The listing builds one solid part. Answer for the finished solid, in the listing's coordinates (mm). Face numbers are marked on the shaded views. Round coordinates to 2 decimals unless told otherwise and drop trailing zeros. Write each loop counter-clockwise with the first axis right and the second up, starting at its lowest first coordinate (ties: lowest second). Pieces come first, ordered by that corner, then holes. Notation, with made-up numbers: (-5, 67) -> (30, 67) arc R28 ccw to (30, 97) -> close; hole circle Ø3 at (-30, 44). An arc over 180 degrees is marked (long way). Write each question's results on one line, items separated by ' | '. Start each with the question number.
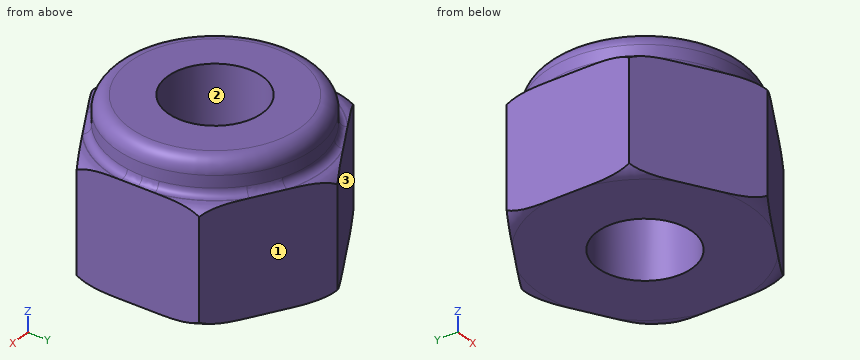
Autodesk Inventor part; units mm, degrees
ref_plane "Work Plane1" through (-12.7, 19.1158, 5.969) normal (-1, 0, 0) x (0, 0, -1)
ref_plane "YZ Plane" through (0, 0, 0) normal (1, 0, 0) x (0, 1, 0)
ref_plane "XZ Plane" through (0, 0, 0) normal (0, 1, 0) x (-1, 0, 0)
sketch "Sketch1" plane through (0, 0, 0) normal (0, 0, 1) x (1, 0, 0)
  line L0 (-12.7, 6.2842) -> (-18.2562, 9.4921)
  line L1 (-18.2562, 9.4921) -> (-18.2563, 15.9079)
  line L2 (-18.2563, 15.9079) -> (-12.7, 19.1158)
  line L3 (-12.7, 19.1158) -> (-7.1438, 15.9079)
  line L4 (-7.1438, 15.9079) -> (-7.1438, 9.4921)
  line L5 (-7.1438, 9.4921) -> (-12.7, 6.2842)
  point P0 (-12.7, 12.7)
  dimension "d0" = 11.1125
extrude "Extrusion1" add sketch "Sketch1" along normal blind 5.969
ref_plane "Work Plane1" through (-12.7, 19.1158, 5.969) normal (-1, 0, 0) x (0, 0, -1)
sketch "Sketch3" plane through (-12.7, 19.1158, 5.969) normal (-1, 0, 0) x (0, 0, -1)
  line L0 (0, 12.8316) -> (5.969, 12.8316)
  line L1 (5.969, 12.8316) -> (5.969, 0)
  line L2 (5.969, 0) -> (0, 0)
  line L3 (0, 0) -> (0, 12.8316)
  line L4 (0, 12.0696) -> (0, 6.4158)
  line L5 (0, 6.4158) -> (5.969, 6.4158)
  line L6 (5.969, 6.4158) -> (5.969, 12.0696)
  arc A0 (5.969, 12.0696) -> (5.625, 12.8316) centre (4.953, 12.0696) ccw
  arc A1 (0.344, 12.8316) -> (0, 12.0696) centre (1.016, 12.0696) ccw
  line L7 (0.344, 12.8316) -> (5.625, 12.8316)
  line L8 (5.969, 12.8316) -> (5.969, 9.6237)
  line L9 (0, 12.8316) -> (0, 9.6237)
  line L10 (0, 9.6237) -> (0, 3.2079)
  dimension "d4" = 1.016
  dimension "d5" = 0.762
  dimension "d6" = 0.762
revolve "Revolution1" cut sketch "Sketch3" angle 360 about axis through (-12.7, 12.7, 5.969) along (0, 0, -1) keep common part contours L0 A0 L1 L5 L3 A1
sketch "Sketch4" plane through (0, 0, 5.969) normal (0, 0, 1) x (1, 0, 0)
  arc A0 (-16.3838, 16.989) -> (-18.2562, 13.7458) centre (-12.7, 12.7) ccw
  circle A1 centre (-12.7, 12.7) radius 5.2451
  dimension "d8" = 10.4902
extrude "Extrusion2" add sketch "Sketch4" along normal blind 1.778
fillet "Fillet1" radius 0.762 1 edges at (-17.9451, 12.7, 7.747)
fillet "Fillet2" radius 0.381 1 edges at (-17.9451, 12.7, 5.969)
hole "Hole1" at (-12.7, 12.7, 7.747) direction (0, 0, -1) diameter 4.9784 end through all
properties part number "HW-00002"
Q1. Find the intervals of material crossed by line 1 (X direction, y = 12.7, z = 4.75); line 2 (Y direction, x = -11, z = 4.25); line 3 (Y direction, x = -16.25, z = 1.5), in increasing order.
Q2. Determine the mould class of the marked faces 1, 2 and 3 for opening direction X: pulls with the +X half, pulls with the -X half, needs draft (parallel to the pull), parting line crosses it, or undercut.
Q3. The part is cut by section B-B, the plane z = 6.5. Write down the section's boundary in (x, y).
Q4. Each of these flat-tipped pins is pushed along its axis until it touches: pin 1 (2 mm diameter, centred on x = -8, y = 9.5, fed in from +Z); pin 2 (4 mm diameter, centred on x = -11.5, z = 6, fed in from +Y). Where does it stop, or does it pass through?
Answers follow:
1) line 1: -18.26 to -15.19, -10.21 to -7.14 | line 2: 7.27 to 10.88, 14.52 to 18.13 | line 3: 8.33 to 17.07
2) face 1: pulls with the +X half | face 2: undercut | face 3: pulls with the -X half
3) outline: circle Ø10.49 at (-12.7, 12.7); hole circle Ø4.98 at (-12.7, 12.7)
4) pin 1: z = 7.72 | pin 2: y = 19.12
